```python
from build123d import *

# Parameters (mm, degrees)
SKETCH2_W           = 50
SKETCH2_H           = 75
SKETCH2_R           = 3
BOSS_EXTRUDE1_DEPTH = 5


with BuildPart() as part:
    # Sketch2 → Boss-Extrude1 (new body)
    with BuildSketch(Plane(origin=(0, 0, 0), x_dir=(1, 0, 0), z_dir=(0, 1, 0))):
        Polygon((-125, 125), (-125, 105), (-95, 105), (-95, 45), (-125, 45), (-125, -45), (-95, -45), (-95, -105), (-125, -105), (-125, -125), (125, -125), (125, -105), (95, -105), (95, -45), (125, -45), (125, 45), (95, 45), (95, 105), (125, 105), (125, 125), align=None)
        with Locations((0, -72.5)):
            Rectangle(SKETCH2_W, SKETCH2_H, mode=Mode.SUBTRACT)
        with Locations((0, 72.5)):
            Rectangle(SKETCH2_W, SKETCH2_H, mode=Mode.SUBTRACT)
        with Locations(Location((-85, 115, 0), (0, 0, 270))):
            Circle(SKETCH2_R, mode=Mode.SUBTRACT)
        with Locations(Location((-85, -115, 0), (0, 0, 270))):
            Circle(SKETCH2_R, mode=Mode.SUBTRACT)
        with Locations(Location((85, 115, 0), (0, 0, 270))):
            Circle(SKETCH2_R, mode=Mode.SUBTRACT)
        with Locations(Location((85, -115, 0), (0, 0, 270))):
            Circle(SKETCH2_R, mode=Mode.SUBTRACT)
    extrude(amount=BOSS_EXTRUDE1_DEPTH)


solid = part.part
```
Model file for the job. Use its own axes, mm. Round coordinates to 2 decimals unless told otherwise and drop trailing zeros. Order: outer loops, then holes, each group sorted by start corner. A loop starts at its lowest first (then second) coordinate and runs counter-clockwise, first axis right, second up. Notation, with made-up numbers: (-16.5, -33) -> (-3.5, -33) arc R26 cw to (-3.5, -7) -> close; hole circle Ø6 at (43.5, 40.25). An arc over 180 degrees is marked (long way). Use one line per item in the form item = value.
Item 1: Cut at D-D, the plane z = 115. Write the cut outline in (x, y), and give its area (3 significant figures).
Returned:
outline = (-125, 0) -> (-88, 0) -> (-88, 5) -> (-125, 5) -> close; (-82, 0) -> (82, 0) -> (82, 5) -> (-82, 5) -> close; (88, 0) -> (125, 0) -> (125, 5) -> (88, 5) -> close
area = 1,190 mm^2
Item 2: Cut at C-C, the plane y = 2.05. Give the number of separate pieces and of enclosed holes in the cut face, and give its area (3 significant figures).
Returned:
separate_pieces = 1
enclosed_holes = 6
area = 47,700 mm^2
Item 3: Cut at B-B, the plane z = -76.5. Write the cut outline in (x, y).
Returned:
outline = (-95, 0) -> (-25, 0) -> (-25, 5) -> (-95, 5) -> close; (25, 0) -> (95, 0) -> (95, 5) -> (25, 5) -> close
Item 4: Flat gauge pins, fed straight in: pin 1 Ø3.5 at (x, z) = (-85, -115) entering from +Y; pin 2 Ø1.5 at (y, z) = (2, 68.5) entering from +X; pin 3 Ø2 at (y, z) = (3.5, -95.5) entering from -X. Where does each tip first touch, or does it go through?
Returned:
pin_1 = through
pin_2 = 95
pin_3 = -95
Item 5: Pull direction Z, two halves, no side cores. Call faces 1 (the face through (-87.662, 2.465, -113.616)), 2 (the face through (-2, 5, -2)): released by +Z, released by -Z, zero draft, split by the parting line, or undercut.
Returned:
face_1 = undercut
face_2 = zero draft
Item 6: Drill centre lines: line 1 (Z direction, x = -110.5, y = 3.45); line 2 (X direction, y = 3.9, z = 115); line 3 (Z direction, x = 18, y = 3.65). Where is each one in solid material? Low to high.
Returned:
line_1 = -125 to -105, -45 to 45, 105 to 125
line_2 = -125 to -88, -82 to 82, 88 to 125
line_3 = -125 to -110, -35 to 35, 110 to 125
Item 7: Cut at A-A, the plane x = -85. Write the cut outline in (y, z), and give its area (3 significant figures).
Returned:
outline = (0, -125) -> (5, -125) -> (5, -118) -> (0, -118) -> close; (0, -112) -> (5, -112) -> (5, 112) -> (0, 112) -> close; (0, 118) -> (5, 118) -> (5, 125) -> (0, 125) -> close
area = 1,190 mm^2
